```python
from build123d import *

# Parameters (mm, degrees)
SKETCH1_W           = 8.2
SKETCH1_H           = 2.88
BOSS_EXTRUDE1_DEPTH = 4.2
SKETCH2_W           = 8.2
SKETCH2_H           = 3.33
BOSS_EXTRUDE2_DEPTH = 0.7
FILLET1_R           = 0.5
FILLET2_R           = 0.3
CUT_EXTRUDE1_DEPTH  = 3
SKETCH4_W           = 0.3
SKETCH4_H           = 0.8
BOSS_EXTRUDE3_DEPTH = 0.7


with BuildPart() as part:
    # Sketch1 → Boss-Extrude1 (new body)
    with BuildSketch(Plane.XY):
        with Locations((4.1, 1.44)):
            Rectangle(SKETCH1_W, SKETCH1_H)
    extrude(amount=BOSS_EXTRUDE1_DEPTH)

    # Sketch2 → Boss-Extrude2 (add)
    with BuildSketch(Plane.XY.offset(4.2)):
        with Locations((4.1, 1.215)):
            Rectangle(SKETCH2_W, SKETCH2_H)
    extrude(amount=BOSS_EXTRUDE2_DEPTH)

    # Fillet1
    fillet1_edges = [part.edges().sort_by_distance(p)[0] for p in [
        (0, 2.88, 2.45),
        (8.2, 2.88, 2.45),
    ]]
    fillet(fillet1_edges, radius=FILLET1_R)

    # Fillet2
    fillet2_edges = [part.edges().sort_by_distance(p)[0] for p in [
        (8.2, -0.45, 4.55),
        (0, -0.45, 4.55),
    ]]
    fillet(fillet2_edges, radius=FILLET2_R)

    # Sketch3 → Cut-Extrude1 (cut)
    with BuildSketch(Plane.XY.offset(4.9)):
        with BuildLine():
            Line((1.266074212, 2.382685956), (6.890517388, 2.382685956))
            ThreePointArc((6.890517388, 2.382685956), (7.173360101, 2.265528668), (7.290517388, 1.982685956))
            Line((7.290517388, 1.982685956), (7.290517388, 1.692784748))
            ThreePointArc((7.290517388, 1.692784748), (7.264361959, 1.550516562), (7.189316204, 1.426853803))
            Line((7.189316204, 1.426853803), (6.63716933, 0.806464056))
            ThreePointArc((6.63716933, 0.806464056), (6.502119746, 0.707448171), (6.338370514, 0.672395002))
            Line((6.338370514, 0.672395002), (1.771767033, 0.672395002))
            ThreePointArc((1.771767033, 0.672395002), (1.610340732, 0.706414744), (1.476372836, 0.802687256))
            Line((1.476372836, 0.802687256), (0.970680014, 1.356541299))
            ThreePointArc((0.970680014, 1.356541299), (0.893141457, 1.481607555), (0.866074212, 1.626249045))
            Line((0.866074212, 1.626249045), (0.866074212, 1.982685956))
            ThreePointArc((0.866074212, 1.982685956), (0.983231499, 2.265528668), (1.266074212, 2.382685956))
        make_face()
    extrude(amount=-CUT_EXTRUDE1_DEPTH, mode=Mode.SUBTRACT)

    # Sketch4 → Boss-Extrude3 (add)
    with BuildSketch(Plane.XZ):
        with Locations((0.49, 2.722)):
            Rectangle(SKETCH4_W, SKETCH4_H)
        with Locations((7.710000038, 2.722)):
            Rectangle(SKETCH4_W, SKETCH4_H)
    extrude(amount=BOSS_EXTRUDE3_DEPTH)


solid = part.part
```
Geometry: final body of the model. Coordinates: model frame, mm. A direction names the side the tool comes from. Round coordinates to 2 decimals unless told otherwise and drop trailing zeros. Loops run counter-clockwise (first coordinate to the right, second up) from the corner with the lowest first, then second, coordinate; pieces in that order, holes last. Notation, with made-up numbers: (12.25, 39) -> (30.25, 39) arc R24 cw to (30.25, 54) -> close; hole circle Ø6 at (-35.75, 52.25). An arc over 180 degrees is marked (long way). Write each question's results on one line, items separated by ' | '.
Item 1: Cut plane A-A on z = 3.35. Return the cut outline in (x, y).
Answers below:
outline: (0, 0) -> (8.2, 0) -> (8.2, 2.38) arc R0.5 ccw to (7.7, 2.88) -> (0.5, 2.88) arc R0.5 ccw to (0, 2.38) -> close; hole (0.87, 1.63) arc R0.4 ccw to (0.97, 1.36) -> (1.48, 0.8) arc R0.4 ccw to (1.77, 0.67) -> (6.34, 0.67) arc R0.4 ccw to (6.64, 0.81) -> (7.19, 1.43) arc R0.4 ccw to (7.29, 1.69) -> (7.29, 1.98) arc R0.4 ccw to (6.89, 2.38) -> (1.27, 2.38) arc R0.4 ccw to (0.87, 1.98) -> close
Item 2: Pin query (flat end, axial travel): pin 1 Ø0.8 at (x, z) = (3.5, 4.5) entering from -Y; pin 2 Ø0.8 at (y, z) = (-0.5, 2.5) entering from +X; pin 3 Ø2 at (x, z) = (3, 2) entering from -Y. Return the tip coordinate at first contact, or that it passes through.
Answers below:
pin 1: stops at y = -0.45 | pin 2: stops at x = 7.86 | pin 3: stops at y = 0
Item 3: Cut plane B-B on y = -0.25. Return the cut outline in (x, z).
Answers below:
outline: (0.02, 4.2) -> (8.18, 4.2) -> (8.18, 4.9) -> (0.02, 4.9) -> close; (0.34, 2.32) -> (0.64, 2.32) -> (0.64, 3.12) -> (0.34, 3.12) -> close; (7.56, 2.32) -> (7.86, 2.32) -> (7.86, 3.12) -> (7.56, 3.12) -> close
Item 4: Cut plane D-D on z = 2.45. Return the cut outline in (x, y).
Answers below:
outline: (0, 0) -> (0.34, 0) -> (0.34, -0.7) -> (0.64, -0.7) -> (0.64, 0) -> (7.56, 0) -> (7.56, -0.7) -> (7.86, -0.7) -> (7.86, 0) -> (8.2, 0) -> (8.2, 2.38) arc R0.5 ccw to (7.7, 2.88) -> (0.5, 2.88) arc R0.5 ccw to (0, 2.38) -> close; hole (0.87, 1.63) arc R0.4 ccw to (0.97, 1.36) -> (1.48, 0.8) arc R0.4 ccw to (1.77, 0.67) -> (6.34, 0.67) arc R0.4 ccw to (6.64, 0.81) -> (7.19, 1.43) arc R0.4 ccw to (7.29, 1.69) -> (7.29, 1.98) arc R0.4 ccw to (6.89, 2.38) -> (1.27, 2.38) arc R0.4 ccw to (0.87, 1.98) -> close
Item 5: Set-up query: faces 5 (the face through (4, 2.383, 3)), 6 (the face through (4, 1, 0)). Return all of +Z, -Z, +X, -X, +Y, -Y with unobstructed straight access to the full face (end or side cutting, diameter ignored); none if empty.
Answers below:
face 5: +Z | face 6: -Z, +X, -X, +Y, -Y
Item 6: Line query: probe 1 along X at (y, z) = (1.75, 2.4); probe 2 along Y at (x, z) = (5.25, 2.35); probe 3 along Z at (x, y) = (6, 2). Output: solid intervals per line, ascending. Write a range as [from, to].
Answers below:
probe 1: x = [0, 0.87], [7.29, 8.2] | probe 2: y = [0, 0.67], [2.38, 2.88] | probe 3: z = [0, 1.9]
Item 7: Cut plane C-C on x = 4.5. Return the cut outline in (y, z), and give its area (3 significant figures).
Answers below:
outline: (-0.45, 4.2) -> (0, 4.2) -> (0, 0) -> (2.88, 0) -> (2.88, 4.9) -> (2.38, 4.9) -> (2.38, 1.9) -> (0.67, 1.9) -> (0.67, 4.9) -> (-0.45, 4.9) -> close | area: 9.30 mm²
Item 8: Pull-direction query (Y, two-part tool) for faces 1 (the face through (4, 2, 1.9)), 2 (the face through (4, 0, 4.9)), 3 (the face through (4, 0.672, 3)), 4 (the face through (4, 2.88, 2)); classes: pulls with the +Y half, pulls with the -Y half, needs draft (parallel to the pull), parting line crosses it, or undercut.
Answers below:
face 1: undercut | face 2: needs draft | face 3: undercut | face 4: pulls with the +Y half
